Verification items for the finished model (mm, model axes). A direction names the side the tool comes from. Round coordinates to 2 decimals unless told otherwise and drop trailing zeros. Loops run counter-clockwise (first coordinate to the right, second up) from the corner with the lowest first, then second, coordinate; pieces in that order, holes last. Notation, with made-up numbers: (-35, -13) -> (9, -13) arc R38 ccw to (9, 26) -> close; hole circle Ø5 at (-26.75, 58). An arc over 180 degrees is marked (long way). Write item = value, one per line. Start each with the question number.
```python
from build123d import *

# Parameters (mm, degrees)
ESQUISSE5_R             = 28
BOSS_EXTRU_5_DEPTH      = 5
ESQUISSE6_R             = 25
ENL_V_MAT_EXTRU_1_DEPTH = 10
ESQUISSE7_W             = 65
ESQUISSE7_H             = 9.382686356
BOSS_EXTRU_6_DEPTH      = 5


with BuildPart() as part:
    # Esquisse5 → Boss.-Extru.5 (new body)
    with BuildSketch(Plane(origin=(0, 5, 0), x_dir=(1, 0, 0), z_dir=(0, 1, 0))):
        with Locations(Location((-36.607266223, 0, 0), (0, 0, 270))):
            Circle(ESQUISSE5_R)
    extrude(amount=-BOSS_EXTRU_5_DEPTH)

    # Esquisse6 → Enlèv. mat.-Extru.1 (cut)
    with BuildSketch(Plane(origin=(0, 5, 0), x_dir=(1, 0, 0), z_dir=(0, 1, 0))):
        with Locations(Location((-36.607266223, 0, 0), (0, 0, 270))):
            Circle(ESQUISSE6_R)
    extrude(amount=-ENL_V_MAT_EXTRU_1_DEPTH, mode=Mode.SUBTRACT)

    # Esquisse7 → Boss.-Extru.6 (add)
    with BuildSketch(Plane(origin=(0, 5, 0), x_dir=(1, 0, 0), z_dir=(0, 1, 0))):
        with Locations((22.754788201, 0)):
            Rectangle(ESQUISSE7_W, ESQUISSE7_H)
    extrude(amount=-BOSS_EXTRU_6_DEPTH)


solid = part.part
```
(1) Scan lines: line 1 (X direction, y = 2.5, z = 0); line 2 (Z direction, x = 44, y = 3.3); line 3 (X direction, y = 3.85, z = -19). Record each from-to range of solid material in increasing order. Write a range as [from, to].
(2) Depth check by flat-ended pin: pin 1 Ø2 at (x, y) = (-22, 1.5) entering from -Z; pin 2 Ø2.5 at (x, y) = (25, 1.5) entering from +Z; pin 3 Ø3 at (x, y) = (-46, 3.5) entering from +Z. Enter the tip coordinate at first touch or a pass-through.
(3) Draft check along Z on faces 1 (the cylindrical face through (-15.5, 2.5, 13.4)), 2 (the cylindrical face through (-64.583, 2.535, -1.165)), 3 (the flat face through (-4, 0, 0)), 4 (the flat face through (23, 3, -4.691)). Enter one of: +Z half, -Z half, draft (parallel to the pull), parting line (faces both ways), or undercut.
(4) Section check D-D on x = 7.5. Enter the section's corners in (y, z), then the cut area to 3 significant figures.
(5) Section check C-C on y = 2.65. Enter the section's corners in (x, z).
(6) Section check A-A on z = 0. Enter the section's corners in (x, y), then the cut area to 3 significant figures.
(7) Section check B-B on x = -55.5. Enter the section's corners in (y, z), then the cut area to 3 significant figures.
(8) Access from +Z, -Z, +X, -X, +Y, -Y to the whole of each face (thin tool, end or side, straight path). Record for faces 5 (the flat face through (-4, 5, 0)), 6 (the flat face through (23, 3, 4.691)).
Computed values:
q1.line_1 = [-64.61, -61.61], [-11.61, 55.25]
q1.line_2 = [-4.69, 4.69]
q1.line_3 = [-57.17, -52.86], [-20.36, -16.04]
q2.pin_1 = -24.47
q2.pin_2 = 4.69
q2.pin_3 = 26.86
q3.face_1 = undercut
q3.face_2 = parting line
q3.face_3 = draft
q3.face_4 = -Z half
q4.outline = (0, -4.69) -> (5, -4.69) -> (5, 4.69) -> (0, 4.69) -> close
q4.area = 46.9 mm²
q5.outline = (-9, -4.69) -> (55.25, -4.69) -> (55.25, 4.69) -> (-9, 4.69) arc R28 ccw (long way) to start; hole circle Ø50 at (-36.61, 0)
q6.outline = (-64.61, 0) -> (-61.61, 0) -> (-61.61, 5) -> (-64.61, 5) -> close; (-11.61, 0) -> (55.25, 0) -> (55.25, 5) -> (-11.61, 5) -> close
q6.area = 349 mm²
q7.outline = (0, -20.67) -> (5, -20.67) -> (5, -16.37) -> (0, -16.37) -> close; (0, 16.37) -> (5, 16.37) -> (5, 20.67) -> (0, 20.67) -> close
q7.area = 42.9 mm²
q8.face_5 = +Z, -Z, +X, -X, +Y
q8.face_6 = +Z, +X, +Y, -Y
